Source: three-view drawing plus pictorial views. Frame: mm from the lowest corner of the part. Round coordinates to 2 decimals unless told otherwise and drop trailing zeros. Loops run counter-clockwise (first coordinate to the right, second up) from the corner with the lowest first, then second, coordinate; pieces in that order, holes last. Notation, with made-up numbers: (33.5, 29.5) -> (38.5, 29.5) arc R13 ccw to (38.5, 44.5) -> close; hole circle Ø9 at (-29.75, 73). An arc over 180 degrees is marked (long way). Answer in a Markdown table with one row per item.
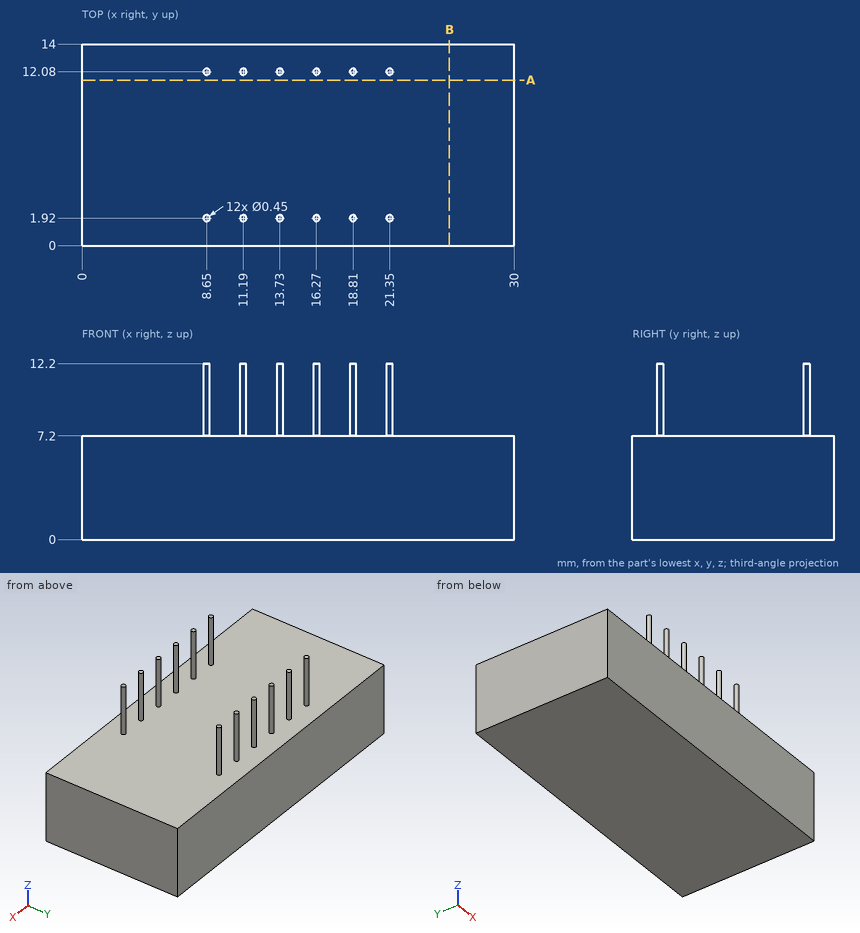
Item 1: Line query: probe 1 along Z at (x, y) = (17.5, 8.25); probe 2 along Y at (x, z) = (11.25, 8.75). Output: solid intervals per line, ascending. Write a range as [from, to].
Answer:
| item | result |
|---|---|
| probe 1 | z = [0, 7.2] |
| probe 2 | y = [1.7, 2.14], [11.86, 12.3] |
Item 2: Pin query (flat end, axial travel): pin 1 Ø3 at (x, z) = (18.5, 5) entering from -Y. Return the tip coordinate at first contact, or that it passes through.
Answer:
| item | result |
|---|---|
| pin 1 | stops at y = 0 |
Item 3: Cut plane B-B (x = 25.5). Output: boundary loops of the cut face in (y, z).
Answer:
| item | result |
|---|---|
| outline | (0, 0) -> (14, 0) -> (14, 7.2) -> (0, 7.2) -> close |
Item 4: Cut plane A-A (y = 11.5). Output: boundary loops of the cut face in (x, z), then the cut area to 3 significant figures.
Answer:
| item | result |
|---|---|
| outline | (0, 0) -> (30, 0) -> (30, 7.2) -> (0, 7.2) -> close |
| area | 216 mm² |
